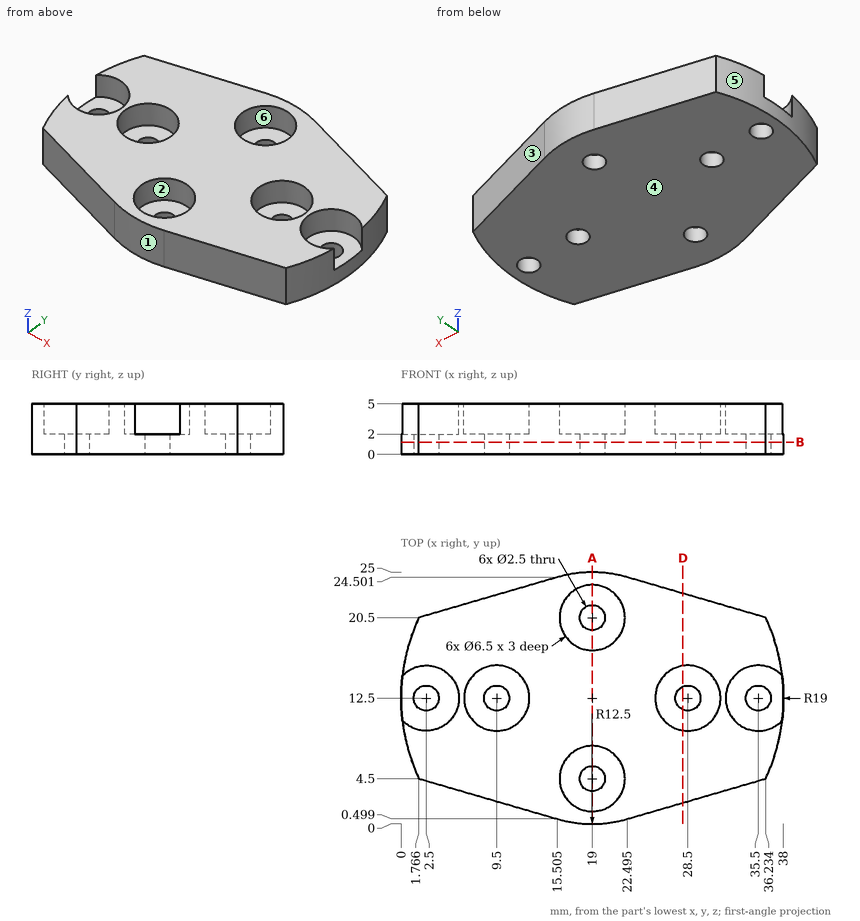
Study the drawing (mm; zero at the part's minimum x, y, z) and answer. A direction names the side the tool comes from. Coordinates: 2 decimals unless noted, no trailing zeros. Write each loop counter-clockwise with the first axis right and the second up, starting at its lowest first coordinate (ties: lowest second). Pieces come first, ordered by that corner, then holes. Notation, with made-up numbers: (-11, -18.5) - (-4, -18.5) arc R20 cw to (-4, -7.5) - close; hole circle Ø2 at (15, -13.75). An arc over 180 degrees is marked (long way). Answer as a JSON object with one key per item and string values.
Q1. Find section A-A (x = 19). Write down the section's boundary in (y, z).
Results list:
{"outline": "(0, 0) - (3.25, 0) - (3.25, 2) - (1.25, 2) - (1.25, 5) - (0, 5) - close; (5.75, 0) - (19.25, 0) - (19.25, 2) - (17.25, 2) - (17.25, 5) - (7.75, 5) - (7.75, 2) - (5.75, 2) - close; (21.75, 0) - (25, 0) - (25, 5) - (23.75, 5) - (23.75, 2) - (21.75, 2) - close"}
Q2. Find section D-D (x = 28). Write down the section's boundary in (y, z) (1 decimal).
Results list:
{"outline": "(2.1, 0) - (11.4, 0) - (11.4, 2) - (9.3, 2) - (9.3, 5) - (2.1, 5) - close; (13.6, 0) - (22.9, 0) - (22.9, 5) - (15.7, 5) - (15.7, 2) - (13.6, 2) - close"}
Q3. Consider L1, parallel to Y at x = 19, z = 0.75; L2, parallel to Y at x = 19, z = 3.3; L3, parallel to X at y = 11.5, z = 4.5. Determine where each line is inside the solid, lowest interval first. Write a range as from..to.
Results list:
{"L1": "y = 0..3.25, 5.75..19.25, 21.75..25", "L2": "y = 0..1.25, 7.75..17.25, 23.75..25", "L3": "x = 5.59..6.41, 12.59..25.41, 31.59..32.41"}
Q4. Given pin 1 Ø4 at (x, y) = (2.5, 12.5) entering from +Z; pin 2 Ø1.5 at (y, z) = (19.5, 4.5) entering from +X; pin 3 Ø1 at (x, z) = (6, 3) entering from -Y, each flat-ended and moving along its own axis, determine where each tip first touches the part or whether it passes through.
Results list:
{"pin 1": "stops at z = 2", "pin 2": "stops at x = 36.94", "pin 3": "stops at y = 3.12"}
Q5. For a pull along Y with two mould halves and no side action, classify the marked faces 1, 2, 3 and 4 as pulls with the +Y half, pulls with the -Y half, needs draft (parallel to the pull), parting line crosses it, or undercut.
Results list:
{"face 1": "pulls with the -Y half", "face 2": "undercut", "face 3": "pulls with the +Y half", "face 4": "needs draft"}
Q6. Which of the six approach directions +Z, -Z, +X, -X, +Y, -Y give full straight-line access (tool end or side, diameter ignored) to the marked faces 5 and 6?
Results list:
{"face 5": "+Z, -Z, -X", "face 6": "+Z"}
Q7. Find section B-B (z = 1.2). State how many separate pieces and enclosed holes the cut face has.
Results list:
{"separate pieces": "1", "enclosed holes": "6"}
